Source: CAD feature listing. Evaluate the final solid. Frame: model axes, mm. A direction names the side the tool comes from. Round coordinates to 2 decimals unless told otherwise and drop trailing zeros. Order: outer loops, then holes, each group sorted by start corner. A loop starts at its lowest first (then second) coordinate and runs counter-clockwise, first axis right, second up.
```python
from build123d import *

# Parameters (mm, degrees)
F0_R      = 5
F1_DEPTH  = 60
F4_DEPTH  = 5
F7_DEPTH  = 5
F8_R      = 2.5
F9_DEPTH  = 12.5
F10_R     = 2.5
F11_DEPTH = 50


with BuildPart() as f1:
    # F0 (on Top) → F1 (new body)
    with BuildSketch(Plane.XY):
        Circle(F0_R)
    extrude(amount=F1_DEPTH)

    # F3 (on offset) → F4 (join)
    with BuildSketch(Plane.XY.offset(8)):
        Polygon((3.175426, 5.5), (-3.175426, 5.5), (-6.350853, 0), (-3.175426, -5.5), (3.175426, -5.5), (6.350853, 0), align=None)
    extrude(amount=F4_DEPTH)

    # F6 (on offset) → F7 (join)
    with BuildSketch(Plane.XY.offset(43)):
        Polygon((3.175426, 5.5), (-3.175426, 5.5), (-6.350853, 0), (-3.175426, -5.5), (3.175426, -5.5), (6.350853, 0), align=None)
    extrude(amount=F7_DEPTH)

    # F8 (on Front) → F9 (cut, symmetric)
    with BuildSketch(Plane.XZ):
        with Locations((0, 54)):
            Circle(F8_R)
    extrude(amount=F9_DEPTH, both=True, mode=Mode.SUBTRACT)

    # F10 (on face) → F11 (cut)
    with BuildSketch(Plane(origin=(0, 0, 0), x_dir=(1, 0, 0), z_dir=(0, 0, -1))):
        Circle(F10_R)
    extrude(amount=-F11_DEPTH, mode=Mode.SUBTRACT)


solid = f1.part
```
1. Section D-D on z = 54. Return loops of the section in (x, y).
2. Access query for faces 1 (the face through (0, -5.5, 45)), 2 (the face through (3, 4, 54)), 3 (the face through (2, 5, 8)), 4 (the face through (-1.08, -4.88, 27.79)), 5 (the face through (2.31, -0.07, 53.04)). Directions: +Z, -Z, +X, -X, +Y, -Y. A direction counts if a zero-diameter tool reaches every point of the face in a straight line with its end or side. Return the directions, or none.
3. Section A-A on x = 0. Return loops of the section in (y, z).
4. Line query: line 1 along Z through (x, y) = (-0.25, 4.25); line 2 along X through (y, z) = (0, 21). Output: solid intervals per line, ascending.
5. First-contact query: pin 1 (2 mm diameter, centred on x = -0.5, y = -0.5, fed in from -Z); pin 2 (5 mm diameter, centred on y = -1.5, z = 18, fed in from +X); pin 3 (6.5 mm diameter, centred on x = 0, z = 54, fed in from -Y); pin 4 (4 mm diameter, centred on x = 3.5, y = 3.5, fed in from -Z). Flat tips, straight axial feed; report the tip coordinate or a pass-through.
6. Section B-B on y = 1. Return loops of the section in (x, z).
7. Section C-C on z = 21.5. Return loops of the section in (x, y), plus the area to 3 significant figures.
8. Pull-direction query (X, two-part tool) for faces 6 (the face through (4.74, -2.79, 45.46)), 7 (the face through (-0.54, 2.44, 24.65)), 8 (the face through (2, 5, 13)); classes: released by +X, released by -X, zero draft, split by the parting line, or undercut.
Result:
1. outline: (-2.5, -4.33) - (-2.5, 4.33) arc R5 ccw to start; (2.5, -4.33) arc R5 ccw to (2.5, 4.33) - close
2. face 1: +Z, -Z, +X, -X, -Y
2. face 2: +Z
2. face 3: -Z
2. face 4: none
2. face 5: +Y, -Y
3. outline: (-5.5, 8) - (-5, 8) - (-5, 0) - (-2.5, 0) - (-2.5, 50) - (2.5, 50) - (2.5, 0) - (5, 0) - (5, 8) - (5.5, 8) - (5.5, 13) - (5, 13) - (5, 43) - (5.5, 43) - (5.5, 48) - (5, 48) - (5, 51.5) - (-5, 51.5) - (-5, 48) - (-5.5, 48) - (-5.5, 43) - (-5, 43) - (-5, 13) - (-5.5, 13) - close; (-5, 56.5) - (5, 56.5) - (5, 60) - (-5, 60) - close
4. line 1: z = 0 to 51.51, 56.49 to 60
4. line 2: x = -5 to -2.5, 2.5 to 5
5. pin 1: stops at z = 50
5. pin 2: stops at x = 5
5. pin 3: stops at y = -5
5. pin 4: stops at z = 0
6. outline: (-5.77, 8) - (-4.9, 8) - (-4.9, 0) - (-2.29, 0) - (-2.29, 50) - (2.29, 50) - (2.29, 0) - (4.9, 0) - (4.9, 8) - (5.77, 8) - (5.77, 13) - (4.9, 13) - (4.9, 43) - (5.77, 43) - (5.77, 48) - (4.9, 48) - (4.9, 60) - (-4.9, 60) - (-4.9, 48) - (-5.77, 48) - (-5.77, 43) - (-4.9, 43) - (-4.9, 13) - (-5.77, 13) - close; hole circle Ø5 at (0, 54)
7. outline: circle Ø10 at (0, 0); hole circle Ø5 at (0, 0)
7. area: 58.9 mm2
8. face 6: released by +X
8. face 7: undercut
8. face 8: zero draft
